from build123d import *

# Parameters (mm, degrees)
SKETCH1_W             = 10
SKETCH1_H             = 40
BOSS_EXTRUDE1_DEPTH   = 10
F_5_0MM_DOWEL_HOLE1_D = 5
FILLET1_R             = 5
CHAMFER1_SIZE         = 5


with BuildPart() as part:
    # Sketch1 → Boss-Extrude1 (new body)
    with BuildSketch(Plane(origin=(0, 0, 0), x_dir=(1, 0, 0), z_dir=(0, 1, 0))):
        Rectangle(SKETCH1_W, SKETCH1_H)
    extrude(amount=BOSS_EXTRUDE1_DEPTH)

    # Ø5.0mm Dowel Hole1 (through all)
    with Locations(Plane(origin=(0, 10, 0), x_dir=(1, 0, 0), z_dir=(0, 1, 0))):
        with Locations((0, 15)):
            Hole(F_5_0MM_DOWEL_HOLE1_D / 2)

    # Fillet1
    fillet1_edges = [part.edges().sort_by_distance(p)[0] for p in [
        (5, 5, -20),
        (-5, 5, -20),
    ]]
    fillet(fillet1_edges, radius=FILLET1_R - 0.0001)  # a hair under: the kernel refuses the full size

    # Chamfer1
    chamfer1_edges = [part.edges().sort_by_distance(p)[0] for p in [
        (0, 0, 20),
    ]]
    chamfer(chamfer1_edges, length=CHAMFER1_SIZE)


solid = part.part
Geometry check sheet. Reference: the model listing, model coordinates, mm. Coordinates: 2 decimals unless noted, no trailing zeros. Loops run counter-clockwise (first coordinate to the right, second up) from the corner with the lowest first, then second, coordinate; pieces in that order, holes last. Notation, with made-up numbers: (-12, 60) - (-7, 60) arc R14 cw to (-7, 70) - close; hole circle Ø11 at (-12, 2). An arc over 180 degrees is marked (long way). Use one line per item in the form item = value. Start each with the question number.
Item 1: Section check B-B, the plane x = -2. Enter the section's corners in (y, z).
Item 2: Section check C-C, the plane z = -15.5. Enter the section's corners in (x, y), and give its area (3 significant figures).
Item 3: Thickness scan on probe 1 along X at (y, z) = (4, -15); probe 2 along Z at (x, y) = (0, 5.25); probe 3 along Z at (x, y) = (2, 5.75). Record the ranges inside material, lowest first.
Item 4: Mould release check, pull along Z, two halves, no side actions. Record for faces 1 (the face through (0.54, 4.93, -12.56)), 2 (the face through (3, 5, -19)), 3 (the face through (0, 0, -3)), 4 (the face through (0, 7, 20)): +Z half, -Z half, draft (parallel to the pull), parting line (faces both ways), or undercut.
Item 5: Gauge pin test, flat ends, axial feed: pin 1 (4.5 mm diameter, centred on x = 0, z = -15, fed in from +Y); pin 2 (3 mm diameter, centred on x = -2, y = 5.5, fed in from -Z). Record the tip position at first contact, or that the pin passes through.
Computed:
q1.outline = (0, -19.58) - (10, -19.58) - (10, -16.5) - (0, -16.5) - close; (0, -13.5) - (10, -13.5) - (10, 20) - (5, 20) - (0, 15) - close
q2.outline = (-4.97, 0) - (-2.45, 0) - (-2.45, 10) - (-4.97, 10) - close; (2.45, 0) - (4.97, 0) - (4.97, 10) - (2.45, 10) - close
q2.area = 50.5 mm2
q3.probe_1 = -5 to -2.5, 2.5 to 5
q3.probe_2 = -20 to -17.5, -12.5 to 20
q3.probe_3 = -19.58 to -16.5, -13.5 to 20
q4.face_1 = undercut
q4.face_2 = -Z half
q4.face_3 = draft
q4.face_4 = +Z half
q5.pin_1 = through
q5.pin_2 = -19.97
